The model under review builds one solid part; all positions refer to its coordinate system, in mm. A direction names the side the tool comes from. Coordinates: 2 decimals unless noted, no trailing zeros. Loops run counter-clockwise (first coordinate to the right, second up) from the corner with the lowest first, then second, coordinate; pieces in that order, holes last. Notation, with made-up numbers: M -9.5,-16.5 L 20.5,-16.5 A12 cw 20.5,-2.5 Z; hole C -12.5,73 d7. An arc over 180 degrees is marked long. One line per item, written item: value.
```python
from build123d import *

# Parameters (mm, degrees)
BOSS_EXTRUDE1_DEPTH = 65
SKETCH2_W           = 5.5
SKETCH2_H           = 2.4
CUT_EXTRUDE1_DEPTH  = 6
LPATTERN1_COUNT     = 3
LPATTERN1_PITCH     = 20
SKETCH3_W           = 6
SKETCH3_H           = 2.4
CUT_EXTRUDE2_DEPTH  = 6
FILLET1_R           = 4
FILLET2_R           = 4
FILLET3_R           = 1
FILLET4_R           = 1


with BuildPart() as part:
    # Sketch1 → Boss-Extrude1 (new body)
    with BuildSketch(Plane.XY):
        Polygon((0, 0), (3.2, 0), (4.2, 0.663324958), (4.2, 3.063324958), (-1, 3.063324958), (-1, 0.663324958), align=None)
    extrude(amount=BOSS_EXTRUDE1_DEPTH)

    # Sketch2 → Cut-Extrude1 (cut)
    with BuildSketch(Plane.ZY.offset(1)):
        with Locations((7.55, 1.863324958)):
            Rectangle(SKETCH2_W, SKETCH2_H)
    cut_extrude1 = extrude(amount=-CUT_EXTRUDE1_DEPTH, mode=Mode.SUBTRACT)

    # LPattern1: Cut-Extrude1 ×3
    with Locations(*[(0, 0, i * LPATTERN1_PITCH) for i in range(1, LPATTERN1_COUNT)]):
        add(cut_extrude1, mode=Mode.SUBTRACT)

    # Sketch3 → Cut-Extrude2 (cut)
    with BuildSketch(Plane.ZY.offset(1)):
        with Locations((58.3, 1.863324958)):
            Rectangle(SKETCH3_W, SKETCH3_H)
    extrude(amount=-CUT_EXTRUDE2_DEPTH, mode=Mode.SUBTRACT)

    # Fillet1
    # the kernel refuses this fillet: 4 mm, written as the material it adds along each edge
    with BuildSketch(Plane(origin=(-1, 0.663324958, 55.3), x_dir=(0, 0, 1), z_dir=(1, 0, 0))) as fillet1_piece_1_section:
        with BuildLine():
            CenterArc((3.666060556, -4), FILLET1_R, 90, 66.421821522)
            Line((0, -2.4), (-0.073321211, -2.368))
            ThreePointArc((-0.073321211, -2.368), (-0.08, -1.2), (-0.08, 0))
            Line((-0.08, 0), (0, 0.08))
            Line((0, 0.08), (3.666060556, 0.08))
            Line((3.666060556, 0.08), (3.666060556, 0))
        make_face()
    fillet1_piece_1 = extrude(amount=5.2, mode=Mode.PRIVATE)
    fillet1_piece_1 = split(fillet1_piece_1, bisect_by=Plane(origin=(0.518931728, -0.344220367, 56.190586237), z_dir=(0.5527707983925672, 0.833333333333333, 0)), keep=Keep.TOP, mode=Mode.PRIVATE)
    fillet1_piece_1 = split(fillet1_piece_1, bisect_by=Plane(origin=(2.681068272, -0.344220367, 56.190586237), z_dir=(-0.5527707983925666, 0.8333333333333335, 0)), keep=Keep.TOP, mode=Mode.PRIVATE)
    add(fillet1_piece_1)

    # Fillet2
    # the kernel refuses this fillet: 4 mm, written as the material it adds along each edge
    with BuildSketch(Plane(origin=(-1, 0.663324958, 61.3), x_dir=(0, 1, 0), z_dir=(1, 0, 0))) as fillet2_piece_1_section:
        with BuildLine():
            CenterArc((4, -3.666060556), FILLET2_R, 113.578178478, 66.421821522)
            Line((0, -3.666060556), (-0.08, -3.666060556))
            Line((-0.08, -3.666060556), (-0.08, 0))
            Line((-0.08, 0), (0, 0.08))
            ThreePointArc((0, 0.08), (1.2, 0.08), (2.368, 0.073321211))
            Line((2.368, 0.073321211), (2.4, 0))
        make_face()
    fillet2_piece_1 = extrude(amount=5.2, mode=Mode.PRIVATE)
    fillet2_piece_1 = split(fillet2_piece_1, bisect_by=Plane(origin=(2.681068272, -0.344220367, 60.409413763), z_dir=(-0.5527707983925666, 0.8333333333333335, 0)), keep=Keep.TOP, mode=Mode.PRIVATE)
    fillet2_piece_1 = split(fillet2_piece_1, bisect_by=Plane(origin=(0.518931728, -0.344220367, 60.409413763), z_dir=(0.5527707983925672, 0.833333333333333, 0)), keep=Keep.TOP, mode=Mode.PRIVATE)
    add(fillet2_piece_1)

    # Fillet3
    fillet3_edges = [part.edges().sort_by_distance(p)[0] for p in [
        (3.2, 0, 32.5),
    ]]
    fillet(fillet3_edges, radius=FILLET3_R)

    # Fillet4
    fillet4_edges = [part.edges().sort_by_distance(p)[0] for p in [
        (0, 0, 32.5),
    ]]
    fillet(fillet4_edges, radius=FILLET4_R)


solid = part.part
```
(1) Add section D-D on z = 47. State the section outline as (x, y) points, then the cut area to 3 significant figures.
Checks:
outline: M -1,0.66 L -0.25,0.17 A1 ccw 0.3,0 L 2.9,0 A1 ccw 3.45,0.17 L 4.2,0.66 Z
area: 2.77 mm^2
(2) Tool access review of faces 3 (the face through (2, 2, 24.8)), 4 (the face through (-1, 1.6, 56.1)): name each direction out of +Z, -Z, +X, -X, +Y, -Y from which nothing blocks a thin tool from reaching the whole face with its end or side.
Checks:
face 3: +X, -X, +Y
face 4: +Z, -Z, -X, +Y, -Y
(3) Add section A-A on y = 2.15. State the section outline as (x, z) points, then the cut area to 3 significant figures.
Checks:
outline: M -1,0 L 4.2,0 L 4.2,4.8 L -1,4.8 Z; M -1,10.3 L 4.2,10.3 L 4.2,24.8 L -1,24.8 Z; M -1,30.3 L 4.2,30.3 L 4.2,44.8 L -1,44.8 Z; M -1,50.3 L 4.2,50.3 L 4.2,55.85 L -1,55.85 Z; M -1,60.75 L 4.2,60.75 L 4.2,65 L -1,65 Z
area: 227 mm^2
(4) Draft analysis for pull direction Z (two halves, no side actions). For faces 1 (the face through (2, 0.663, 28)), 2 (the face through (2, 3.063, 53)), state which applies: pulls with the +Z half, pulls with the -Z half, needs draft (parallel to the pull), parting line crosses it, or undercut.
Checks:
face 1: undercut
face 2: needs draft
(5) To check wall thickness, follow L1, parallel to Z at x = 0, y = 2.75; L2, parallel to Z at x = 2.15, y = 1.5; L3, parallel to Y at x = 3.05, z = 30. State the ranges of each line that lie inside material, in increasing order. Write a range as [from, to].
Checks:
L1: [0, 4.8], [10.3, 24.8], [30.3, 44.8], [50.3, 55.45], [61.15, 65]
L2: [0, 4.8], [10.3, 24.8], [30.3, 44.8], [50.3, 56.52], [60.08, 65]
L3: [0.01, 0.66]
(6) Add section C-C on x = 1.45. State the section outline as (y, z) points, then the cut area to 3 significant figures.
Checks:
outline: M 0,0 L 3.06,0 L 3.06,4.8 L 0.66,4.8 L 0.66,10.3 L 3.06,10.3 L 3.06,24.8 L 0.66,24.8 L 0.66,30.3 L 3.06,30.3 L 3.06,44.8 L 0.66,44.8 L 0.66,50.3 L 3.06,50.3 L 3.06,55.3 A4 cw 0.72,58.3 A4 cw 3.06,61.3 L 3.06,65 L 0,65 Z
area: 150 mm^2
(7) Add section B-B on z = 23. State the section outline as (x, y) points, then the cut area to 3 significant figures.
Checks:
outline: M -1,0.66 L -0.25,0.17 A1 ccw 0.3,0 L 2.9,0 A1 ccw 3.45,0.17 L 4.2,0.66 L 4.2,3.06 L -1,3.06 Z
area: 15.2 mm^2
